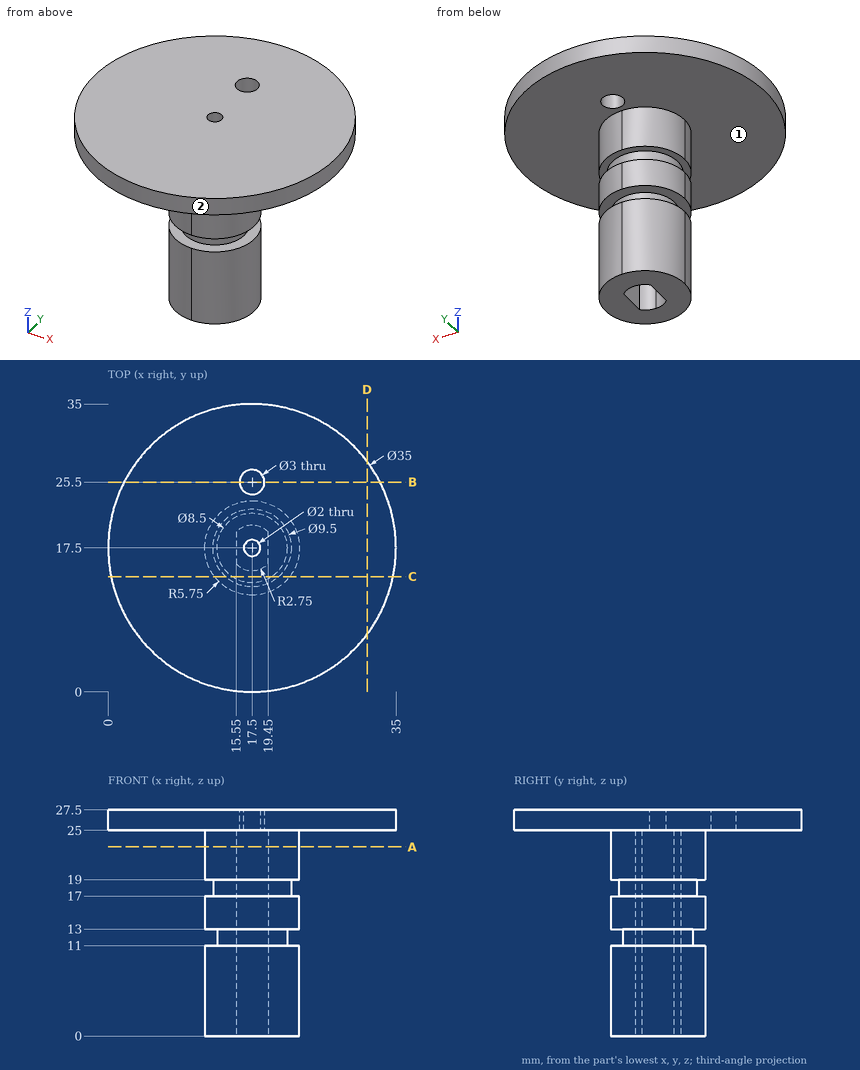
Check sheet for the drawn part. Datum: minimum x, y, z corner. Units: mm. A direction names the side the tool comes from. Round coordinates to 2 decimals unless told otherwise and drop trailing zeros. Order: outer loops, then holes, each group sorted by start corner. A loop starts at its lowest first (then second) coordinate and runs counter-clockwise, first axis right, second up. Notation, with made-up numbers: (17.5, -0.5) -> (24.5, -0.5) arc R28 cw to (24.5, 19.5) -> close; hole circle Ø7 at (72.25, 65.25). An arc over 180 degrees is marked (long way). Return JSON: item names as keys, results as strings. Group by question number.
Q1. Section check D-D, the plane x = 31.5. Record the boundary of the cut face in (y, z).
Q2. Tool access check on the marked faces 1 and 2. Record the directions out of +Z, -Z, +X, -X, +Y, -Y that give a thin tool (end or side, any length) a straight path to the whole face; none if there is none.
Q3. Section check B-B, the plane y = 25.5. Record the boundary of the cut face in (x, z), plus the area to 3 significant figures.
Q4. Section check A-A, the plane z = 23. Record the boundary of the cut face in (x, y), plus the area to 3 significant figures.
Q5. Gauge pin test, flat ends, axial feed: pin 1 (1.8 mm diameter, centred on x = 17.5, y = 25.5, fed in from -Z); pin 2 (8 mm diameter, centred on y = 24.5, z = 7.5, fed in from +X); pin 3 (3 mm diameter, centred on y = 18, z = 10.5, fed in from -X); pin 4 (4.5 mm diameter, centred on y = 18.5, z = 15.5, fed in from +X). Record the tip position at first contact, or that the pin passes through.
Q6. Material ranges on probe 1 along Y at (x, z) = (17.5, 27.05); probe 2 along X at (y, z) = (17.5, 14.5); probe 3 along X at (y, z) = (16, 3.25), recorded low to high. Write a range as from..to.
Q7. Section check C-C, the plane y = 14. Record the boundary of the cut face in (x, z), plus the area to 3 significant figures.
Numbers:
{
 "1": {"outline": "(7, 25) -> (28, 25) -> (28, 27.5) -> (7, 27.5) -> close"},
 "2": {"face 1": "-Z", "face 2": "+Z, -Z"},
 "3": {"outline": "(1.94, 25) -> (16, 25) -> (16, 27.5) -> (1.94, 27.5) -> close; (19, 25) -> (33.06, 25) -> (33.06, 27.5) -> (19, 27.5) -> close", "area": "70.3 mm^2"},
 "4": {"outline": "circle Ø11.5 at (17.5, 17.5); hole (15.55, 15.56) arc R2.75 ccw to (19.45, 15.56) -> (19.45, 19.44) arc R2.75 ccw to (15.55, 19.44) -> close", "area": "84.4 mm^2"},
 "5": {"pin 1": "through", "pin 2": "x = 22.41", "pin 3": "x = 11.75", "pin 4": "x = 23.25"},
 "6": {"probe 1": "0..16.5, 18.5..24, 27..35", "probe 2": "11.75..15.55, 19.45..23.25", "probe 3": "11.95..15.55, 19.45..23.05"},
 "7": {"outline": "(0.35, 25) -> (12.94, 25) -> (12.94, 19) -> (14.29, 19) -> (14.29, 17) -> (12.94, 17) -> (12.94, 13) -> (15.09, 13) -> (15.09, 11) -> (12.94, 11) -> (12.94, 0) -> (22.06, 0) -> (22.06, 11) -> (19.91, 11) -> (19.91, 13) -> (22.06, 13) -> (22.06, 17) -> (20.71, 17) -> (20.71, 19) -> (22.06, 19) -> (22.06, 25) -> (34.65, 25) -> (34.65, 27.5) -> (0.35, 27.5) -> close", "area": "300 mm^2"}
}
